Source: CAD feature listing. Evaluate the final solid. Frame: model axes, mm. Face numbers are marked on the shaded views. Round coordinates to 2 decimals unless told otherwise and drop trailing zeros. Write each loop counter-clockwise with the first axis right and the second up, starting at its lowest first coordinate (ties: lowest second). Pieces come first, ordered by that corner, then holes. Notation, with made-up numbers: (-13.5, 4.25) - (42.5, 4.25) arc R13 cw to (42.5, 16.25) - close; hole circle Ø4 at (58.5, 67.5). An arc over 180 degrees is marked (long way). Write item = value, one per line. Start each with the question number.
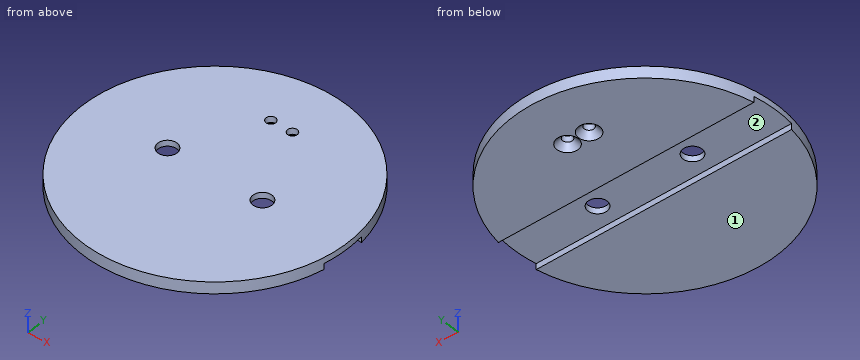
```python
from build123d import *

# Parameters (mm, degrees)
ESBO_O1_R                                           = 90
FLANGE_BASE2_DEPTH                                  = 8
CORTE_EXTRUS_O3_START                               = -4
CORTE_EXTRUS_O3_DEPTH                               = 4
ESBO_O13_R                                          = 6.5
CORTE_EXTRUS_O4_DEPTH                               = 4
ESCAREADO_PARA_PARAFUSO_ALLEN_SEXTAVADO_D           = 6.6
ESCAREADO_PARA_PARAFUSO_ALLEN_SEXTAVADO_CSINK_D     = 14.44
ESCAREADO_PARA_PARAFUSO_ALLEN_SEXTAVADO_CSINK_ANGLE = 90


# Sheet-metal steps are written as plain solids
with BuildPart() as part:
    # Esboço1 → Flange-base2 (new body)
    with BuildSketch(Plane.XY):
        Circle(ESBO_O1_R)
    extrude(amount=-FLANGE_BASE2_DEPTH)

    # Esboço12 → Corte-extrusão3 (cut)
    with BuildSketch(Plane(origin=(0, 0, -8), x_dir=(-1, 0, 0), z_dir=(0, 0, -1)).offset(CORTE_EXTRUS_O3_START)):
        with BuildLine():
            Line((-88.741196746, 15), (88.741196746, 15))
            ThreePointArc((88.741196746, 15), (90, 0), (88.741196746, -15))
            Line((88.741196746, -15), (-88.741196746, -15))
            ThreePointArc((-88.741196746, -15), (-90, 0), (-88.741196746, 15))
        make_face()
    extrude(amount=CORTE_EXTRUS_O3_DEPTH, mode=Mode.SUBTRACT)

    # Esboço13 → Corte-extrusão4 (cut)
    with BuildSketch(Plane(origin=(0, 0, -4), x_dir=(-1, 0, 0), z_dir=(0, 0, -1))):
        with Locations((33, 0)):
            Circle(ESBO_O13_R)
        with Locations((-33, 0)):
            Circle(ESBO_O13_R)
    extrude(amount=-CORTE_EXTRUS_O4_DEPTH, mode=Mode.SUBTRACT)

    # Escareado para parafuso Allen sextavado escareado de M63 (through all)
    with Locations(Plane(origin=(0, 0, -8), x_dir=(-1, 0, 0), z_dir=(0, 0, -1))):
        with Locations((-7.5, 53), (7.5, 53)):
            CounterSinkHole(ESCAREADO_PARA_PARAFUSO_ALLEN_SEXTAVADO_D / 2, ESCAREADO_PARA_PARAFUSO_ALLEN_SEXTAVADO_CSINK_D / 2, counter_sink_angle=ESCAREADO_PARA_PARAFUSO_ALLEN_SEXTAVADO_CSINK_ANGLE)


solid = part.part
```
(1) Ray query, L1, parallel to X at y = 53, z = -3.2; L2, parallel to Y at x = -5, z = -6.75; L3, parallel to Z at x = -5, y = -12. Return the intervals inside material, ascending. Write a range as from..to.
(2) Section C-C (x = -33). Return the cut outline in (y, z), plus the area to 3 significant figures.
(3) Section B-B (y = 53). Return the cut outline in (x, z), plus the area to 3 significant figures.
(4) Section A-A (z = -5.75). Return the cut outline in (x, y).
(5) Section D-D (x = -78.5). Return the cut outline in (y, z), plus the area to 3 significant figures.
(6) Contact query for flat-ended pins moving along their axis: P1, Ø2, axis at x = -57, y = -52.5, coming from the +Z side; P2, Ø2, axis at x = 29, z = -7, coming from the +Y side; P3, Ø1.2, axis at x = 7, z = -7, coming from the -Y side; P4, Ø4, axis at y = 46, z = -5, coming from the +X side. Output: stop coordinate, or through.
(7) Pull-direction query (Y, two-part tool) for the marked faces 1 and 2; classes: +Y half, -Y half, draft (parallel to the pull), parting line (faces both ways), or undercut.
Solution:
q1.L1 = -72.74..-10.8, -4.2..4.2, 10.8..72.74
q1.L2 = -89.86..-15, 15..47.58, 58.42..89.86
q1.L3 = -4..0
q2.outline = (-83.73, -8) - (-15, -8) - (-15, -4) - (-6.5, -4) - (-6.5, 0) - (-83.73, 0) - close; (6.5, -4) - (15, -4) - (15, -8) - (83.73, -8) - (83.73, 0) - (6.5, 0) - close
q2.area = 1,170 mm^2
q3.outline = (-72.74, -8) - (-14.72, -8) - (-10.8, -4.08) - (-10.8, 0) - (-72.74, 0) - close; (-4.2, -4.08) - (-0.28, -8) - (0.28, -8) - (4.2, -4.08) - (4.2, 0) - (-4.2, 0) - close; (10.8, -4.08) - (14.72, -8) - (72.74, -8) - (72.74, 0) - (10.8, 0) - close
q3.area = 1,030 mm^2
q4.outline = (-88.74, -15) arc R90 ccw to (88.74, -15) - close; (-88.74, 15) - (88.74, 15) arc R90 ccw to start; hole circle Ø9.94 at (-7.5, 53); hole circle Ø9.94 at (7.5, 53)
q5.outline = (-44.02, -8) - (-15, -8) - (-15, -4) - (15, -4) - (15, -8) - (44.02, -8) - (44.02, 0) - (-44.02, 0) - close
q5.area = 584 mm^2
q6.P1 = 0
q6.P2 = 85.53
q6.P3 = -89.77
q6.P4 = 78.51
q7.face_1 = draft
q7.face_2 = undercut
